Source: CAD feature listing. Evaluate the final solid. Frame: model axes, mm. A direction names the side the tool comes from. Coordinates: 2 decimals unless noted, no trailing zeros. One line per item, written item: value. Start each with the question number.
1. Access query for faces 1 (the flat face through (-3, 22.225, -43)), 2 (the cylindrical face through (136.18, -0.24, -133.21)). Directions: +Z, -Z, +X, -X, +Y, -Y. A direction counts if a zero-diameter tool reaches every point of the face in a straight line with its end or side. Return the directions, or none.
2. Mould query, pull axis Z, two halves, no side actions, for faces 3 (the cylindrical face through (-45.426, -0.24, -204.567)), 4 (the flat face through (-1, -22.225, -14)), 5 (the cylindrical face through (-35.524, -0.24, 36.314)). Classes: released by +Z, released by -Z, zero draft, split by the parting line, or undercut.
3. Line query: line 1 (X direction, y = -11, z = 85.5); line 2 (Z direction, x = -60, y = 2); line 3 (X direction, y = -5, z = 153). Output: solid intervals per line, ascending.
4. First-contact query: P1, Ø3, axis at y = -7, z = -160, coming from the +X side; P2, Ø2, axis at x = -48.5, y = 6.5, coming from the -Z side; P3, Ø3, axis at y = -9, z = 41, coming from the +X side. Flat tips, straight axial feed; report the tip coordinate or a pass-through.
from build123d import *

# Parameters (mm, degrees)
F0_R     = 209.55
F1_DEPTH = 22.225
F3_R     = 5.08


# Not quite as in the source:
# - a feature of the source that left no trace in its solid (it failed there, or was rolled back) is left out


with BuildPart() as f1:
    # F0 (on Front) → F1 (new body, symmetric)
    with BuildSketch(Plane.XZ):
        Circle(F0_R)
        with BuildLine():
            ThreePointArc((0, 190.5), (134.703841816, 134.703841816), (190.5, 0))
            ThreePointArc((190.5, 0), (134.703841816, -134.703841816), (0, -190.5))
            ThreePointArc((0, -190.5), (-134.703841816, -134.703841816), (-190.5, 0))
            ThreePointArc((-190.5, 0), (-134.703841816, 134.703841816), (0, 190.5))
        make_face(mode=Mode.SUBTRACT)
        with BuildLine():
            ThreePointArc((0, -50.8), (35.9210244843, -35.9210244843), (50.8, 0))
            ThreePointArc((50.8, 0), (35.9210244843, 35.9210244843), (0, 50.8))
            ThreePointArc((0, 50.8), (-35.9210244843, 35.9210244843), (-50.8, 0))
            ThreePointArc((-50.8, 0), (-35.9210244843, -35.9210244843), (0, -50.8))
        make_face()
        with BuildLine():
            ThreePointArc((0, 7.62), (5.3881536726, 5.3881536726), (7.62, 0))
            ThreePointArc((7.62, 0), (-5.3881536726, -5.3881536726), (0, 7.62))
        make_face(mode=Mode.SUBTRACT)
        with BuildLine():
            Line((0, -190.5), (0, -50.8))
            ThreePointArc((0, -50.8), (-35.9210244843, -35.9210244843), (-50.8, 0))
            Line((-50.8, 0), (-190.5, 0))
            ThreePointArc((-190.5, 0), (-134.703841816, -134.703841816), (0, -190.5))
        make_face()
        with BuildLine():
            ThreePointArc((0, 50.8), (35.9210244843, 35.9210244843), (50.8, 0))
            Line((50.8, 0), (190.5, 0))
            ThreePointArc((190.5, 0), (134.703841816, 134.703841816), (0, 190.5))
            Line((0, 190.5), (0, 50.8))
        make_face()
    extrude(amount=F1_DEPTH, both=True)

    # F3
    f3_edges = [f1.edges().sort_by_distance(p)[0] for p in [
        (0, -22.225, -120.65),
        (0, 22.225, -120.65),
        (120.65, -22.225, 0),
        (-120.65, -22.225, 0),
        (0, -22.225, 120.65),
        (-209.55, 22.225, 0),
        (-209.55, -22.225, 0),
        (-134.703842, -22.225, 134.703842),
        (-35.921024, -22.225, 35.921024),
        (134.703842, -22.225, -134.703842),
        (35.921024, -22.225, -35.921024),
        (120.65, 22.225, 0),
        (134.703842, 22.225, -134.703842),
        (-120.65, 22.225, 0),
        (-35.921024, 22.225, 35.921024),
        (0, 22.225, 120.65),
    ]]
    fillet(f3_edges, radius=F3_R)


solid = f1.part
Computed values:
1. face 1: +Z, -Z, +X, -X, +Y
1. face 2: +Y, -Y
2. face 3: split by the parting line
2. face 4: zero draft
2. face 5: undercut
3. line 1: x = -191.31 to -170.24, 0 to 191.31
3. line 2: z = -200.78 to 0, 180.8 to 200.78
3. line 3: x = -143.19 to -113.5, 0 to 143.19
4. P1: stops at x = 137.07
4. P2: stops at z = -204.1
4. P3: stops at x = 205.79
